```python
from build123d import *

# Parameters (mm, degrees)
BOSS_EXTRUDE1_DEPTH = 25.4
CUT_EXTRUDE3_START  = -3.175
CUT_EXTRUDE3_DEPTH  = 19.05
SKETCH5_R           = 3.175
CUT_EXTRUDE4_DEPTH  = 6.35
CUT_EXTRUDE5_REACH  = 62.685
SKETCH6_R           = 6.4135


with BuildPart() as part:
    # Sketch1 → Boss-Extrude1 (new body)
    with BuildSketch(Plane(origin=(0, 0, 0), x_dir=(1, 0, 0), z_dir=(0, 1, 0))):
        with BuildLine():
            Line((26, 22.525), (31.75, 22.525))
            Line((31.75, 22.525), (31.75, -22.525))
            Line((31.75, -22.525), (-31.75, -22.525))
            Line((-31.75, -22.525), (-31.75, 22.525))
            Line((-31.75, 22.525), (-26, 22.525))
            ThreePointArc((-26, 22.525), (0, -3.475), (26, 22.525))
        make_face()
    extrude(amount=BOSS_EXTRUDE1_DEPTH)

    # Sketch3 → Cut-Extrude3 (cut)
    with BuildSketch(Plane(origin=(0, 25.4, 0), x_dir=(1, 0, 0), z_dir=(0, 1, 0)).offset(CUT_EXTRUDE3_START)):
        with BuildLine():
            Line((-31.75, -16.175), (31.75, -16.175))
            Line((31.75, -16.175), (31.75, 22.525))
            Line((31.75, 22.525), (29.175, 22.525))
            ThreePointArc((29.175, 22.525), (0, -6.65), (-29.175, 22.525))
            Line((-29.175, 22.525), (-31.75, 22.525))
            Line((-31.75, 22.525), (-31.75, -16.175))
        make_face()
    extrude(amount=-CUT_EXTRUDE3_DEPTH, mode=Mode.SUBTRACT)

    # Sketch5 → Cut-Extrude4 (cut)
    with BuildSketch(Plane.XY.offset(22.525)):
        with Locations((-19.05, 12.7)):
            Circle(SKETCH5_R)
        with Locations((19.05, 12.7)):
            Circle(SKETCH5_R)
    extrude(amount=-CUT_EXTRUDE4_DEPTH, mode=Mode.SUBTRACT)

    # Cut-Extrude5: up to this face of the body (flat: up to its plane)
    cut_extrude5_end = Plane(part.part.faces().sort_by_distance((0, 12.7, 16.175))[0])
    # Sketch6 → Cut-Extrude5 (cut, up to the picked face)
    with BuildSketch(Plane(origin=(0, 0, -22.525), x_dir=(-1, 0, 0), z_dir=(0, 0, -1)), mode=Mode.PRIVATE) as cut_extrude5_sk1:
        with Locations((-19.05, 12.7)):
            Circle(SKETCH6_R)
    cut_extrude5_tool1 = split(extrude(cut_extrude5_sk1.sketch, amount=-CUT_EXTRUDE5_REACH, mode=Mode.PRIVATE), bisect_by=cut_extrude5_end, keep=Keep.BOTH, mode=Mode.PRIVATE)
    # Sketch6 → Cut-Extrude5 (cut, up to the picked face)
    with BuildSketch(Plane(origin=(0, 0, -22.525), x_dir=(-1, 0, 0), z_dir=(0, 0, -1)), mode=Mode.PRIVATE) as cut_extrude5_sk2:
        with Locations((19.05, 12.7)):
            Circle(SKETCH6_R)
    cut_extrude5_tool2 = split(extrude(cut_extrude5_sk2.sketch, amount=-CUT_EXTRUDE5_REACH, mode=Mode.PRIVATE), bisect_by=cut_extrude5_end, keep=Keep.BOTH, mode=Mode.PRIVATE)
    add(cut_extrude5_tool1.solids().sort_by(Axis((19.05, 12.7, -22.525), (0, 0, 1)))[0], mode=Mode.SUBTRACT)
    add(cut_extrude5_tool2.solids().sort_by(Axis((-19.05, 12.7, -22.525), (0, 0, 1)))[0], mode=Mode.SUBTRACT)


solid = part.part
```
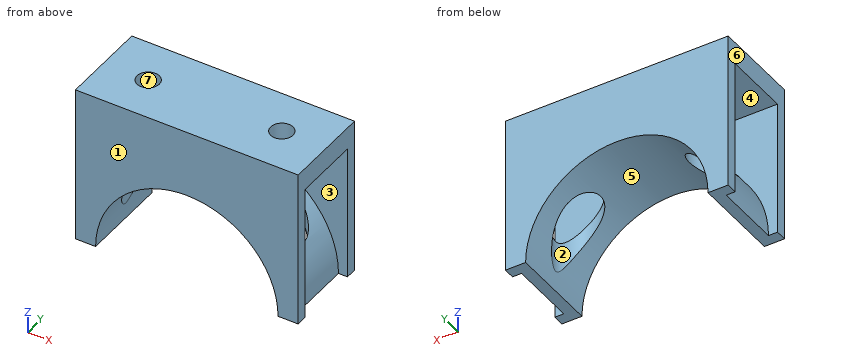
Build history of the part. All positions in model axes, mm. Face numbers are marked on the shaded views. A direction names the side the tool comes from. Round coordinates to 2 decimals unless told otherwise and drop trailing zeros. Order: outer loops, then holes, each group sorted by start corner. A loop starts at its lowest first (then second) coordinate and runs counter-clockwise, first axis right, second up. Notation, with made-up numbers: (-25, 19) -> (-21, 19) arc R23 cw to (-21, 28) -> close; hole circle Ø7 at (53.25, 12.25). An arc over 180 degrees is marked (long way). Answer in a Markdown table with one row per item.
1) Band-saw the part on A-A on x = 0. Give the cut face in (y, z) (3 decimals).
Values:
| item | result |
|---|---|
| outline | (0, 3.475) -> (25.4, 3.475) -> (25.4, 22.525) -> (0, 22.525) -> close; hole (3.175, 6.65) -> (22.225, 6.65) -> (22.225, 16.175) -> (3.175, 16.175) -> close |
2) Band-saw the part on B-B on z = 10. Give the cut face in (x, y) (3 decimals), and give its area (3 significant figures).
Values:
| item | result |
|---|---|
| outline | (-31.75, 0) -> (31.75, 0) -> (31.75, 3.175) -> (-31.75, 3.175) -> close; (-31.75, 22.225) -> (31.75, 22.225) -> (31.75, 25.4) -> (-31.75, 25.4) -> close |
| area | 403 mm2 |
3) Pin check, flat tips, straight feed: P1, Ø10, axis at x = -18, y = 15.5, coming from the +Z side (3 decimals); P2, Ø1.5, axis at x = -14.5, y = 18.5, coming from the -Z side; P3, Ø7.5, axis at x = 19.05, y = 12.7, coming from the -Z side (3 decimals); P4, Ø5.5, axis at x = -4.5, y = 16.5, coming from the -Z side. Stop position of each tip, or through.
Values:
| item | result |
|---|---|
| P1 | z = 22.525 |
| P2 | z = -1.47 |
| P3 | z = 16.175 |
| P4 | z = 2.44 |
4) Wall check: L1, parallel to Y at x = -19, z = -3; L2, parallel to Y at x = -10, z = 8 (3 decimals); L3, parallel to X at y = 12.7, z = -10.5. Give the ranges that are in metal, low to high.
Values:
| item | result |
|---|---|
| L1 | 0 to 6.29, 19.11 to 25.4 |
| L2 | 0 to 3.175, 22.225 to 25.4 |
| L3 | -26.58 to -25.46, 25.46 to 26.58 |
5) Mould opens along X. For the marked faces 4, 5, 6 and 7 say: released by +X, released by -X, zero draft, split by the parting line, or undercut.
Values:
| item | result |
|---|---|
| face 4 | zero draft |
| face 5 | undercut |
| face 6 | released by -X |
| face 7 | undercut |
6) Band-saw the part on C-C on y = 12.7. Give the number of separate pieces and of enclosed holes in the cut face, and give its area (3 significant figures).
Values:
| item | result |
|---|---|
| separate pieces | 6 |
| enclosed holes | 0 |
| area | 474 mm2 |
7) Which spindle directions (+Z, -Z, +X, -X, +Y, -Y) get a long thin tool onto all of the face, cutting with end or side? Do the marked faces 1, 2 and 3. Say none if no direction does.
Values:
| item | result |
|---|---|
| face 1 | +Z, -Z, +X, -X, -Y |
| face 2 | -Z |
| face 3 | none |
